Build history of the part. All positions in model axes, mm. A direction names the side the tool comes from. Round coordinates to 2 decimals unless told otherwise and drop trailing zeros. One line per question, with ' | ' between items.
from build123d import *

# Parameters (mm, degrees)
IZIM1_W                     = 15
IZIM1_H                     = 15
Y_KSEKLIK_EKSTR_ZYON1_DEPTH = 150


with BuildPart() as part:
    # Çizim1 → Yükseklik-Ekstrüzyon1 (new body, symmetric)
    with BuildSketch(Plane.XY):
        Rectangle(IZIM1_W, IZIM1_H)
    extrude(amount=Y_KSEKLIK_EKSTR_ZYON1_DEPTH, both=True)

    # Çizim3 → M8 Dişli Delik1 (revolve, cut)
    with BuildSketch(Plane(origin=(0, 0, 150), x_dir=(0, -1, 0), z_dir=(1, 0, 0))):
        Polygon((0, 0), (0, 24.292926105), (3.4, 22.25), (3.4, 0), align=None)
    m8_di_li_delik1 = revolve(axis=Axis((0, 0, 156.35), (0, 0, -1)), mode=Mode.SUBTRACT)

    # Aynalama1: M8 Dişli Delik1 across plane
    add(m8_di_li_delik1.mirror(Plane.XY), mode=Mode.SUBTRACT)


solid = part.part
(1) 3-axis set-ups, long thin cutter, end or side, ignore diameter. For faces 5 (the cylindrical face through (3.32, 0.74, -139.03)), 6 (the cylindrical face through (3.32, 0.74, 139.03)), 7 (the flat face through (0, 7.5, 2)): which of +Z, -Z, +X, -X, +Y, -Y reach the whole face in a straight line?
Calculated:
face 5: -Z | face 6: +Z | face 7: +Z, -Z, +X, -X, +Y
(2) Mould opens along X. For faces 1 (the flat face through (-7.5, 0, 2)), 2 (the flat face through (-2, 3, 150)), 3 (the flat face through (7.5, 0, 2)), 4 (the conical face through (0.359, 0.469, -126.062)) say: pulls with the +X half, pulls with the -X half, needs draft (parallel to the pull), parting line crosses it, or undercut.
Calculated:
face 1: pulls with the -X half | face 2: needs draft | face 3: pulls with the +X half | face 4: undercut
(3) Wall check: line 1 (Y direction, x = 0, z = 137.75); line 2 (Y direction, x = 2, z = 137.5). Give the ranges that are in metal, low to high. Write a range as from..to.
Calculated:
line 1: -7.5..-3.4, 3.4..7.5 | line 2: -7.5..-2.75, 2.75..7.5
(4) Drop flat-ended pins along their axis: pin 1 (5.5 mm diameter, centred on x = 0, y = 0, fed in from -Z); pin 2 (8 mm diameter, centred on x = 0, y = 0, fed in from +Z). Give the stop position or say it passes through.
Calculated:
pin 1: z = -127.36 | pin 2: z = 150
